Read the model definition and answer for the solid it produces. Units are mm, in the model's axes. Face numbers are marked on the shaded views. Coordinates: 2 decimals unless noted, no trailing zeros. Write each loop counter-clockwise with the first axis right and the second up, starting at its lowest first coordinate (ties: lowest second). Pieces come first, ordered by that corner, then holes. Notation, with made-up numbers: (-19.75, 10) - (-6.75, 10) arc R16 ccw to (-6.75, 30) - close; hole circle Ø5 at (30.5, -1.5). An arc over 180 degrees is marked (long way). Use a Markdown table: item, result.
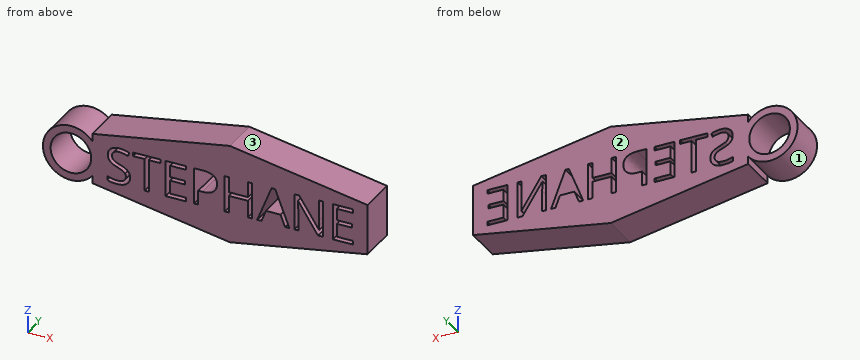
from build123d import *

# Parameters (mm, degrees)
F0_R     = 8
F1_DEPTH = 15


with BuildPart() as f1:
    # F0 (on Front) → F1 (new body)
    with BuildSketch(Plane.XZ):
        Polygon((-21.752604651, 34.6147342483), (-75.9170310667, 25.0640844767), (-75.9170310667, 22.1353372474), (-75.9170310667, 15.0640844767), (-75.9170310667, 7.992831706), (-75.9170310667, 5.0640844767), (-21.752604651, -4.486565295), (32.4118217647, 5.0640844767), (32.4118217647, 25.0640844767), align=None)
        with BuildLine():
            add(Edge.make_bspline(
                [(-61.8588756487, 13.6911544495), (-61.0137733992, 12.770932), (-61.0137733992, 11.3060881009)],
                knots=[0, 0, 0, 1, 1, 1], degree=2))
            add(Edge.make_bspline(
                [(-61.0137733992, 11.3060881009), (-61.0137733992, 9.4186930769), (-62.3831520442, 8.3607502609)],
                knots=[0, 0, 0, 1, 1, 1], degree=2))
            add(Edge.make_bspline(
                [(-62.3831520442, 8.3607502609), (-63.7525306893, 7.3028074448), (-66.1000369379, 7.3028074448)],
                knots=[0, 0, 0, 1, 1, 1], degree=2))
            add(Edge.make_bspline(
                [(-66.1000369379, 7.3028074448), (-68.6416037031, 7.3028074448), (-70.0125473523, 7.9601091945)],
                knots=[0, 0, 0, 1, 1, 1], degree=2))
            Line((-70.0125473523, 7.9601091945), (-70.0125473523, 9.5626734602))
            add(Edge.make_bspline(
                [(-70.0125473523, 9.5626734602), (-69.1298850028, 9.1933324771), (-68.0938522451, 8.9773619022)],
                knots=[0, 0, 0, 1, 1, 1], degree=2))
            add(Edge.make_bspline(
                [(-68.0938522451, 8.9773619022), (-67.0578194874, 8.7613913273), (-66.0405667796, 8.7613913273)],
                knots=[0, 0, 0, 1, 1, 1], degree=2))
            add(Edge.make_bspline(
                [(-66.0405667796, 8.7613913273), (-64.3785323556, 8.7613913273), (-63.5365601144, 9.3920880061)],
                knots=[0, 0, 0, 1, 1, 1], degree=2))
            add(Edge.make_bspline(
                [(-63.5365601144, 9.3920880061), (-62.6945878732, 10.0227846849), (-62.6945878732, 11.1495876843)],
                knots=[0, 0, 0, 1, 1, 1], degree=2))
            add(Edge.make_bspline(
                [(-62.6945878732, 11.1495876843), (-62.6945878732, 11.8913996589), (-62.9935036689, 12.3655959211)],
                knots=[0, 0, 0, 1, 1, 1], degree=2))
            add(Edge.make_bspline(
                [(-62.9935036689, 12.3655959211), (-63.2924194645, 12.8397921833), (-63.9919763266, 13.2419982539)],
                knots=[0, 0, 0, 1, 1, 1], degree=2))
            add(Edge.make_bspline(
                [(-63.9919763266, 13.2419982539), (-64.6915331887, 13.6442043245), (-66.1188169879, 14.1512656742)],
                knots=[0, 0, 0, 1, 1, 1], degree=2))
            add(Edge.make_bspline(
                [(-66.1188169879, 14.1512656742), (-68.1126322951, 14.8649075738), (-68.9686895738, 15.8430351774)],
                knots=[0, 0, 0, 1, 1, 1], degree=2))
            add(Edge.make_bspline(
                [(-68.9686895738, 15.8430351774), (-69.8247468524, 16.821162781), (-69.8247468524, 18.3955569718)],
                knots=[0, 0, 0, 1, 1, 1], degree=2))
            add(Edge.make_bspline(
                [(-69.8247468524, 18.3955569718), (-69.8247468524, 20.0482013708), (-68.583698549, 21.0263289744)],
                knots=[0, 0, 0, 1, 1, 1], degree=2))
            add(Edge.make_bspline(
                [(-68.583698549, 21.0263289744), (-67.3426502455, 22.004456578), (-65.2956247967, 22.004456578)],
                knots=[0, 0, 0, 1, 1, 1], degree=2))
            add(Edge.make_bspline(
                [(-65.2956247967, 22.004456578), (-63.1640891229, 22.004456578), (-61.3737243573, 21.2219544952)],
                knots=[0, 0, 0, 1, 1, 1], degree=2))
            Line((-61.3737243573, 21.2219544952), (-61.8933057403, 19.775890646))
            add(Edge.make_bspline(
                [(-61.8933057403, 19.775890646), (-63.664890456, 20.5177026206), (-65.336314905, 20.5177026206)],
                knots=[0, 0, 0, 1, 1, 1], degree=2))
            add(Edge.make_bspline(
                [(-65.336314905, 20.5177026206), (-66.6571784209, 20.5177026206), (-67.4005553997, 19.9511711126)],
                knots=[0, 0, 0, 1, 1, 1], degree=2))
            add(Edge.make_bspline(
                [(-67.4005553997, 19.9511711126), (-68.1439323784, 19.3846396045), (-68.1439323784, 18.3767769218)],
                knots=[0, 0, 0, 1, 1, 1], degree=2))
            add(Edge.make_bspline(
                [(-68.1439323784, 18.3767769218), (-68.1439323784, 17.6349649472), (-67.8700566494, 17.1592036808)],
                knots=[0, 0, 0, 1, 1, 1], degree=2))
            add(Edge.make_bspline(
                [(-67.8700566494, 17.1592036808), (-67.5961809204, 16.6834424144), (-66.9451391874, 16.2874963605)],
                knots=[0, 0, 0, 1, 1, 1], degree=2))
            add(Edge.make_bspline(
                [(-66.9451391874, 16.2874963605), (-66.2940974545, 15.8915503066), (-64.9544538886, 15.4126590318)],
                knots=[0, 0, 0, 1, 1, 1], degree=2))
            add(Edge.make_bspline(
                [(-64.9544538886, 15.4126590318), (-62.7039778982, 14.611376899), (-61.8588756487, 13.6911544495)],
                knots=[0, 0, 0, 1, 1, 1], degree=2))
        make_face(mode=Mode.SUBTRACT)
        Polygon((-53.6864238951, 20.323642104), (-53.6864238951, 7.4999979697), (-55.3484583191, 7.4999979697), (-55.3484583191, 20.323642104), (-59.8775803748, 20.323642104), (-59.8775803748, 21.8010060365), (-49.1573018393, 21.8010060365), (-49.1573018393, 20.323642104), align=None, mode=Mode.SUBTRACT)
        Polygon((-39.0317248868, 8.9867519272), (-39.0317248868, 7.4999979697), (-47.0038561072, 7.4999979697), (-47.0038561072, 21.8010060365), (-39.0317248868, 21.8010060365), (-39.0317248868, 20.323642104), (-45.3418216832, 20.323642104), (-45.3418216832, 15.71626984), (-39.4135859033, 15.71626984), (-39.4135859033, 14.2482959325), (-45.3418216832, 14.2482959325), (-45.3418216832, 8.9867519272), align=None, mode=Mode.SUBTRACT)
        with BuildLine():
            add(Edge.make_bspline(
                [(-32.1550965825, 21.8010060365), (-26.7965223189, 21.8010060365), (-26.7965223189, 17.6349649472)],
                knots=[0, 0, 0, 1, 1, 1], degree=2))
            add(Edge.make_bspline(
                [(-26.7965223189, 17.6349649472), (-26.7965223189, 15.4627391651), (-28.2785812638, 14.2936810533)],
                knots=[0, 0, 0, 1, 1, 1], degree=2))
            add(Edge.make_bspline(
                [(-28.2785812638, 14.2936810533), (-29.7606402088, 13.1246229415), (-32.5181775489, 13.1246229415)],
                knots=[0, 0, 0, 1, 1, 1], degree=2))
            Line((-32.5181775489, 13.1246229415), (-34.2021220313, 13.1246229415))
            Line((-34.2021220313, 13.1246229415), (-34.2021220313, 7.4999979697))
            Line((-34.2021220313, 7.4999979697), (-35.8641564553, 7.4999979697))
            Line((-35.8641564553, 7.4999979697), (-35.8641564553, 21.8010060365))
            Line((-35.8641564553, 21.8010060365), (-32.1550965825, 21.8010060365))
        make_face(mode=Mode.SUBTRACT)
        Polygon((-12.9462354518, 21.8010060365), (-12.9462354518, 7.4999979697), (-14.6082698759, 7.4999979697), (-14.6082698759, 14.2295158825), (-22.1421999299, 14.2295158825), (-22.1421999299, 7.4999979697), (-23.8042343539, 7.4999979697), (-23.8042343539, 21.8010060365), (-22.1421999299, 21.8010060365), (-22.1421999299, 15.71626984), (-14.6082698759, 15.71626984), (-14.6082698759, 21.8010060365), align=None, mode=Mode.SUBTRACT)
        Polygon((1.6865534981, 7.4999979697), (-0.0349510843, 7.4999979697), (-1.8159258249, 12.0479000754), (-7.5469710799, 12.0479000754), (-9.3060357623, 7.4999979697), (-10.9899802446, 7.4999979697), (-5.3371851979, 21.8604761948), (-3.9380714737, 21.8604761948), align=None, mode=Mode.SUBTRACT)
        with BuildLine():
            Line((14.8231984655, 21.8010060365), (14.8231984655, 7.4999979697))
            Line((14.8231984655, 7.4999979697), (12.9264134166, 7.4999979697))
            Line((12.9264134166, 7.4999979697), (5.1107826128, 19.5004499128))
            Line((5.1107826128, 19.5004499128), (5.0325324045, 19.5004499128))
            add(Edge.make_bspline(
                [(5.0325324045, 19.5004499128), (5.1890328211, 17.387694289), (5.1890328211, 15.6286296067)],
                knots=[0, 0, 0, 1, 1, 1], degree=2))
            Line((5.1890328211, 15.6286296067), (5.1890328211, 7.4999979697))
            Line((5.1890328211, 7.4999979697), (3.6521987303, 7.4999979697))
            Line((3.6521987303, 7.4999979697), (3.6521987303, 21.8010060365))
            Line((3.6521987303, 21.8010060365), (5.5302037292, 21.8010060365))
            Line((5.5302037292, 21.8010060365), (13.327054483, 9.8475042184))
            Line((13.327054483, 9.8475042184), (13.4053046913, 9.8475042184))
            add(Edge.make_bspline(
                [(13.4053046913, 9.8475042184), (13.3865246413, 10.1104249182), (13.317664458, 11.5439687341)],
                knots=[0, 0, 0, 1, 1, 1], degree=2))
            add(Edge.make_bspline(
                [(13.317664458, 11.5439687341), (13.2488042748, 12.9775125499), (13.2675843247, 13.5941241912)],
                knots=[0, 0, 0, 1, 1, 1], degree=2))
            Line((13.2675843247, 13.5941241912), (13.2675843247, 21.8010060365))
            Line((13.2675843247, 21.8010060365), (14.8231984655, 21.8010060365))
        make_face(mode=Mode.SUBTRACT)
        Polygon((26.7266201503, 8.9867519272), (26.7266201503, 7.4999979697), (18.7544889299, 7.4999979697), (18.7544889299, 21.8010060365), (26.7266201503, 21.8010060365), (26.7266201503, 20.323642104), (20.416523354, 20.323642104), (20.416523354, 15.71626984), (26.3447591339, 15.71626984), (26.3447591339, 14.2482959325), (20.416523354, 14.2482959325), (20.416523354, 8.9867519272), align=None, mode=Mode.SUBTRACT)
        with BuildLine():
            Line((-75.9170310667, 15.0640844767), (-75.9170310667, 22.1353372474))
            ThreePointArc((-75.9170310667, 22.1353372474), (-95.3430256224, 15.0640844767), (-75.9170310667, 7.992831706))
            Line((-75.9170310667, 7.992831706), (-75.9170310667, 15.0640844767))
        make_face()
        with Locations((-84.3430256224, 15.0640844767)):
            Circle(F0_R, mode=Mode.SUBTRACT)
    extrude(amount=F1_DEPTH)


solid = f1.part
(1) Each of these flat-tipped pins is pushed along its axis until it touches: P1, Ø0.8, axis at x = 14, y = -4.5, coming from the -Z side; P2, Ø1, axis at x = -62, y = -11, coming from the -Z side; P3, Ø1.6, axis at y = -5.5, z = 8, coming from the -X side; P4, Ø4, axis at x = -20, y = -10, coming from the -Z side. Where does it stop, or does it pass through?
Report:
| item | result |
|---|---|
| P1 | stops at z = 1.75 |
| P2 | stops at z = 2.52 |
| P3 | stops at x = -93.39 |
| P4 | stops at z = -4.49 |
(2) The mould has two halves that part along X. Classify the marked faces 1, 2 and 3: pulls with the +X half, pulls with the -X half, needs draft (parallel to the pull), parting line crosses it, or undercut.
Report:
| item | result |
|---|---|
| face 1 | undercut |
| face 2 | needs draft |
| face 3 | pulls with the +X half |
(3) A cutting plane is placed at A-A, the plane x = -18. Write down the section's boundary in (y, z).
Report:
| item | result |
|---|---|
| outline | (-15, -3.82) - (0, -3.82) - (0, 14.23) - (-15, 14.23) - close; (-15, 15.72) - (0, 15.72) - (0, 33.95) - (-15, 33.95) - close |
(4) A cutting plane is placed at C-C, the plane z = -0.5. Write down the section's boundary in (x, y), and give its area (3 significant figures).
Report:
| item | result |
|---|---|
| outline | (-44.36, -15) - (0.86, -15) - (0.86, 0) - (-44.36, 0) - close |
| area | 678 mm² |
(5) A cutting plane is placed at B-B, the plane x = 9. Write down the section's boundary in (y, z), and give its area (3 significant figures).
Report:
| item | result |
|---|---|
| outline | (-15, 0.94) - (0, 0.94) - (0, 13.53) - (-15, 13.53) - close; (-15, 16.48) - (0, 16.48) - (0, 29.19) - (-15, 29.19) - close |
| area | 380 mm² |
(6) A cutting plane is placed at D-D, the plane y = -3.25. Count the separate pieces of the cut face and the enclosed holes in it, and give its area (3 significant figures).
Report:
| item | result |
|---|---|
| separate pieces | 1 |
| enclosed holes | 9 |
| area | 2,900 mm² |
(7) Straight lines are drawn through the part: L1, parallel to Z at x = -44, y = -8; L2, parallel to Z at x = -68.5, y = -4; L3, parallel to Z at x = -27.5, y = -10. For each, find the intervals that lie inside material, in ascending order.
Report:
| item | result |
|---|---|
| L1 | z = -0.56 to 7.5, 8.99 to 14.25, 15.72 to 20.32, 21.8 to 30.69 |
| L2 | z = 3.76 to 7.49, 9.07 to 15.4, 21.09 to 26.37 |
| L3 | z = -3.47 to 15.12, 20.11 to 33.6 |
